Design review of the part shown in the three views and the two pictorial views. Dimensions are in mm from the part's minimum x, y and z. A direction names the side the tool comes from. Round coordinates to 2 decimals unless told otherwise and drop trailing zeros. Loops run counter-clockwise (first coordinate to the right, second up) from the corner with the lowest first, then second, coordinate; pieces in that order, holes last. Notation, with made-up numbers: (-39.75, 57) -> (-24.75, 57) arc R5 cw to (-24.75, 61) -> close; hole circle Ø2 at (-32, -33). An arc over 180 degrees is marked (long way). One line per question, with ' | ' between items. Start each with the question number.
1. For pin 1 Ø0.8 at (y, z) = (3.5, 7) entering from +X; pin 2 Ø1.6 at (y, z) = (3, 4) entering from -X; pin 3 Ø3 at (x, z) = (15, 3) entering from -Y; pin 4 Ø3 at (x, z) = (18.5, 5) entering from +Y, all flat-tipped, find the tip position at first contact; note any pin that passes through.
2. For the marked faces 1, 2 and 3, list the 3-axis set-ups (+Z, -Z, +X, -X, +Y, -Y) from which the entire face can be reached by the end or side of a thin tool; tool diameter is ignored.
3. Consider section D-D (z = 2). Write out the cut boundary in (x, y), and give its area (3 significant figures).
4. Consider section C-C (x = 18.5). Write out the cut boundary in (y, z).
5. Consider section A-A (z = 5). Write out the cut boundary in (x, y).
6. Consider section B-B (y = 5.5). Write out the cut boundary in (x, z), and give its area (3 significant figures).
7. Wall thickness on line 1 along Z through (x, y) = (18.5, 5.15); line 2 along X through (y, z) = (5.6, 5); line 3 along X through (y, z) = (5.25, 5): over which ranges is each line inside the solid? List them lowest first.
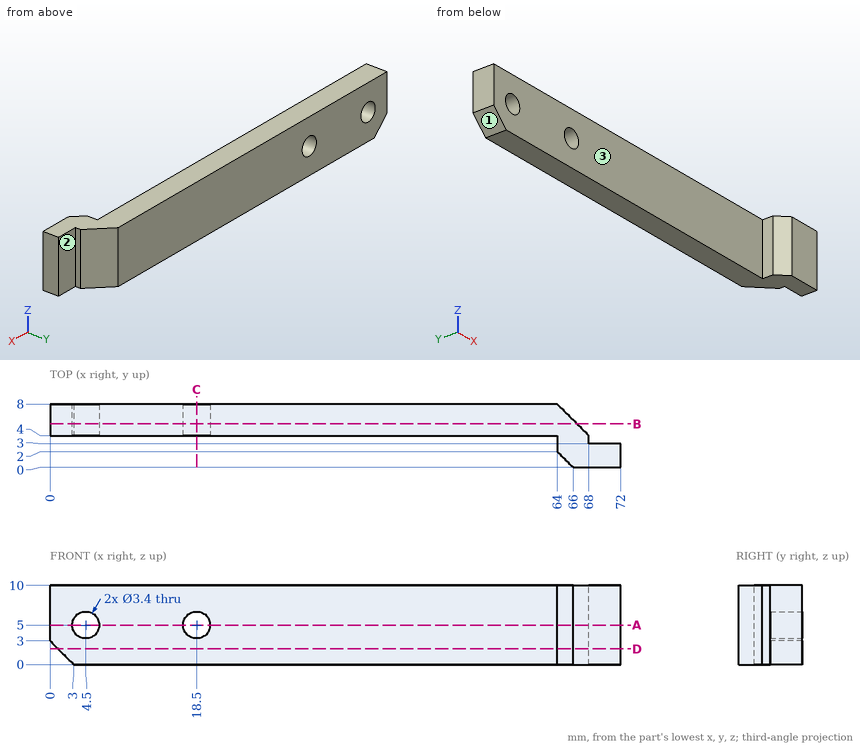
Answer block:
1) pin 1: stops at x = 68 | pin 2: stops at x = 64 | pin 3: stops at y = 4 | pin 4: passes through
2) face 1: -Z, -X, +Y, -Y | face 2: +Z, -Z, +X, +Y | face 3: +Z, -Z, -X, -Y
3) outline: (1, 4) -> (64, 4) -> (64, 2) -> (66, 0) -> (72, 0) -> (72, 3) -> (68, 3) -> (68, 4) -> (64, 8) -> (1, 8) -> close | area: 286 mm2
4) outline: (4, 0) -> (8, 0) -> (8, 3.3) -> (4, 3.3) -> close; (4, 6.7) -> (8, 6.7) -> (8, 10) -> (4, 10) -> close
5) outline: (0, 4) -> (2.8, 4) -> (2.8, 8) -> (0, 8) -> close; (6.2, 4) -> (16.8, 4) -> (16.8, 8) -> (6.2, 8) -> close; (20.2, 4) -> (64, 4) -> (64, 2) -> (66, 0) -> (72, 0) -> (72, 3) -> (68, 3) -> (68, 4) -> (64, 8) -> (20.2, 8) -> close
6) outline: (0, 3) -> (3, 0) -> (66.5, 0) -> (66.5, 10) -> (0, 10) -> close; hole circle Ø3.4 at (4.5, 5); hole circle Ø3.4 at (18.5, 5) | area: 642 mm2
7) line 1: z = 0 to 3.3, 6.7 to 10 | line 2: x = 0 to 2.8, 6.2 to 16.8, 20.2 to 66.4 | line 3: x = 0 to 2.8, 6.2 to 16.8, 20.2 to 66.75
